Geometry: final body of the model. Coordinates: model frame, mm. A direction names the side the tool comes from. Coordinates: 2 decimals unless noted, no trailing zeros. Write each loop counter-clockwise with the first axis right and the second up, starting at its lowest first coordinate (ties: lowest second). Pieces come first, ordered by that corner, then holes. Notation, with made-up numbers: (20, 74.5) -> (60, 74.5) arc R26 ccw to (60, 99.5) -> close; hole circle Ø5 at (17.5, 13). An arc over 180 degrees is marked (long way). One line per item, written item: value.
Autodesk Inventor part; units mm, degrees
ref_plane "YZ Plane" through (0, 0, 0) normal (1, 0, 0) x (0, 1, 0)
ref_plane "XZ Plane" through (0, 0, 0) normal (0, 1, 0) x (-1, 0, 0)
ref_plane "XY Plane" through (0, 0, 0) normal (0, 0, 1) x (1, 0, 0)
sketch "Sketch1" plane through (0, 0, 0) normal (0, 1, 0) x (-1, 0, 0)
  line L0 (0, 0) -> (0, -15) construction
  line L1 (-9, 0) -> (-9, -15)
  line L2 (9, -15) -> (9, 0)
  arc A0 (9, 0) -> (-9, 0) centre (0, 0) ccw
  arc A1 (-9, -15) -> (9, -15) centre (0, -15) ccw
  line L3 (0, 0) -> (0, -15) construction
  line L4 (-8, 0) -> (-8, -15)
  line L5 (8, -15) -> (8, 0)
  arc A2 (8, 0) -> (-8, 0) centre (0, 0) ccw
  arc A3 (-8, -15) -> (8, -15) centre (0, -15) ccw
  point P0 (0, -7.5)
  point P1 (0, -7.5)
  dimension "d0" = 15
  dimension "d1" = 18
  dimension "d2" = 15
  dimension "d3" = 16
extrude "Extrusion1" add sketch "Sketch1" along normal blind 3
sketch "Sketch2" plane through (0, 3, 0) normal (0, 1, 0) x (1, 0, 0)
  line L0 (0, 0) -> (0, 15) construction
  line L1 (12.5, 0) -> (12.5, 15)
  line L2 (-12.5, 15) -> (-12.5, 0)
  arc A0 (-12.5, 0) -> (12.5, 0) centre (0, 0) ccw
  arc A1 (12.5, 15) -> (-12.5, 15) centre (0, 15) ccw
  line L3 (0, 0) -> (0, 15) construction
  line L4 (8, 0) -> (8, 15)
  line L5 (-8, 15) -> (-8, 0)
  arc A2 (-8, 0) -> (8, 0) centre (0, 0) ccw
  arc A3 (8, 15) -> (-8, 15) centre (0, 15) ccw
  point P0 (0, 7.5)
  point P1 (0, 7.5)
  dimension "d6" = 15
  dimension "d7" = 25
  dimension "d8" = 15
  dimension "d9" = 16
extrude "Extrusion2" add sketch "Sketch2" along normal mid plane 1.5
fillet "Fillet1" radius 1.5 4 edges at (0, 3.75, -23) (8, 3.75, -7.5) (0, 3.75, 8) (-8, 3.75, -7.5)
properties part number "Spacer"
(1) Section D-D (x = -10.5). Return the cut outline in (y, z), then the cut area to 3 significant figures.
Responses:
outline: (2.25, -21.78) -> (3.75, -21.78) -> (3.75, 6.78) -> (2.25, 6.78) -> close
area: 42.8 mm2
(2) Reachability of faces 5 (the flat face through (-9, 1, -8)), 6 (the cylindrical face through (0, 1, -23)), 7 (the cylindrical face through (-8.43, 3.3, -7.4)), 8 (the flat face through (9, 1, -7)) from +Z, -Z, +X, -X, +Y, -Y: full face, straight path, thin tool, end or side. Return the list, or none.
Responses:
face 5: +Z, -Z, -X, -Y
face 6: +Y, -Y
face 7: +Y
face 8: +Z, -Z, +X, -Y
(3) Section A-A (z = -7). Return the cut outline in (x, y), then the cut area to 3 significant figures.
Responses:
outline: (-12.5, 2.25) -> (-9, 2.25) -> (-9, 0) -> (-8, 0) -> (-8, 2.25) arc R1.5 ccw to (-9.5, 3.75) -> (-12.5, 3.75) -> close; (8, 0) -> (9, 0) -> (9, 2.25) -> (12.5, 2.25) -> (12.5, 3.75) -> (9.5, 3.75) arc R1.5 ccw to (8, 2.25) -> close
area: 17.0 mm2
(4) Section B-B (y = 0.55). Return the cut outline in (x, z).
Responses:
outline: (-9, -15) arc R9 ccw to (9, -15) -> (9, 0) arc R9 ccw to (-9, 0) -> close; hole (-8, -15) arc R8 ccw to (8, -15) -> (8, 0) arc R8 ccw to (-8, 0) -> close
(5) Pull-direction query (X, two-part tool) for faces 1 (the flat face through (-8, 1, -8)), 2 (the cylindrical face through (0, 1, 9)), 3 (the flat face through (-9.3, 2.25, -9.1)), 4 (the flat face through (-12.5, 3, -8)); classes: released by +X, released by -X, zero draft, split by the parting line, or undercut.
Responses:
face 1: undercut
face 2: split by the parting line
face 3: zero draft
face 4: released by -X
(6) First-contact query: pin 1 (1.1 mm diameter, centred on y = 1, z = -8, fed in from -X); pin 2 (1.8 mm diameter, centred on y = 1, z = -7.5, fed in from +X); pin 3 (2 mm diameter, centred on x = -7.5, z = 1.5, fed in from +Y); pin 4 (5 mm diameter, centred on x = 2.5, z = 7.5, fed in from -Y). Flat tips, straight axial feed; report the tip coordinate or a pass-through.
Responses:
pin 1: stops at x = -9
pin 2: stops at x = 9
pin 3: stops at y = 3.48
pin 4: stops at y = 0
(7) Line query: line 1 (X direction, y = 0.5, z = -6); line 2 (Z direction, x = 3, y = 1.75); line 3 (X direction, y = 2.4, z = 3). Output: solid intervals per line, ascending. Write a range as [from, to].
Responses:
line 1: x = [-9, -8], [8, 9]
line 2: z = [-23.49, -22.42], [7.42, 8.49]
line 3: x = [-12.13, -7.42], [7.42, 12.13]
(8) Section C-C (x = 0). Return the cut outline in (y, z), then the cut area to 3 significant figures.
Responses:
outline: (0, -24) -> (2.25, -24) -> (2.25, -27.5) -> (3.75, -27.5) -> (3.75, -24.5) arc R1.5 ccw to (2.25, -23) -> (0, -23) -> close; (0, 8) -> (2.25, 8) arc R1.5 ccw to (3.75, 9.5) -> (3.75, 12.5) -> (2.25, 12.5) -> (2.25, 9) -> (0, 9) -> close
area: 17.0 mm2
